Verification items for the finished model (mm, model axes). A direction names the side the tool comes from. Coordinates: 2 decimals unless noted, no trailing zeros. Order: outer loops, then holes, each group sorted by start corner. A loop starts at its lowest first (then second) coordinate and runs counter-clockwise, first axis right, second up. Notation, with made-up numbers: (-13, 3.5) -> (18, 3.5) arc R27 cw to (18, 26.5) -> close; hole circle Ø2 at (19, 27). An arc over 180 degrees is marked (long way). Use CSV: the item, a comma, the result in double quotes. Start each with the question number.
1) Sectioned sample at B-B on z = -66. Record the boundary of the cut face in (x, y) (3 decimals).
2) Tool access check on faces 4 (the cylindrical face through (2.52, 1.93, -47.08)), 5 (the cylindrical face through (-0.069, -1.567, -88.386)), 6 (the flat face through (0, 0, -2.381)). Record the directions out of +Z, -Z, +X, -X, +Y, -Y that give a thin tool (end or side, any length) a straight path to the whole face; none if there is none.
3) Scan lines: line 1 along Z through (x, y) = (3, -2.25); line 2 along Y through (x, z) = (0.25, -23); line 3 along Z through (x, y) = (-0.5, 1.25). Record each from-to range of solid material in increasing order.
4) Go/stop test with flat-tipped pins: pin 1 (0.5 mm diameter, centred on y = -0.5, z = -1, fed in from -X); pin 2 (3 mm diameter, centred on x = -1.5, y = 1.5, fed in from -Z); pin 3 (1 mm diameter, centred on y = 3, z = -62, fed in from -X); pin 4 (1 mm diameter, centred on y = -2.5, z = -83, fed in from -X). Record where each tip stops, or that it passes through.
5) Release check for a two-part mould opening along Y. For faces 1 (the cylindrical face through (-2.302, 0.725, -93.105)), 2 (the flat face through (0.8, 1.37, -1.17)), 3 (the flat face through (0.1, 3.1, -4.763)) record: released by +Y, released by -Y, zero draft, split by the parting line, or undercut.
from build123d import *

# Parameters (mm, degrees)
SKETCH12_R          = 2.413
BOSS_EXTRUDE1_DEPTH = 9.525
CHAMFER1_SIZE       = 0.60325
CHAMFER2_SIZE       = 0.3095625
FILLET1_R           = 0.264583333
CUT_EXTRUDE2_DEPTH  = 2.38125


with BuildPart() as part:
    # Sketch13 → Revolve1 (revolve)
    with BuildSketch(Plane(origin=(0, 0, 0), x_dir=(0, 0, -1), z_dir=(1, 0, 0)), mode=Mode.PRIVATE) as revolve1_sk:
        Polygon((0, 0), (0, 4.7625), (4.7625, 4.7625), (4.7625, 2.936875), (5.715, 2.936875), (5.953125, 3.175), (87.074375, 3.175), (87.3125, 2.936875), (87.3125, 0), align=None)
    revolve(revolve1_sk.sketch.rotate(Axis((0, 0, -87.3125), (0, 0, 1)), 90), axis=Axis((0, 0, -87.3125), (0, 0, 1)))

    # Sketch12 → Boss-Extrude1 (add)
    with BuildSketch(Plane(origin=(0, 0, -87.3125), x_dir=(-1, 0, 0), z_dir=(0, 0, -1))):
        Circle(SKETCH12_R)
    extrude(amount=BOSS_EXTRUDE1_DEPTH)

    # Sketch5 → Cut-Revolve1 (revolve, cut)
    with BuildSketch(Plane(origin=(0, 0, 0), x_dir=(0, 0, -1), z_dir=(1, 0, 0))):
        Polygon((87.3125, 2.413), (90.06205, 2.413), (89.2175, 1.56845), (87.3125, 1.56845), align=None)
    revolve(axis=Axis((0, 0, -87.3125), (0, 0, 1)), mode=Mode.SUBTRACT)

    # Chamfer1
    chamfer1_edges = [part.edges().sort_by_distance(p)[0] for p in [
        (2.413, 0, -96.8375),
    ]]
    chamfer(chamfer1_edges, length=CHAMFER1_SIZE)

    # Chamfer2
    chamfer2_edges = [part.edges().sort_by_distance(p)[0] for p in [
        (4.7625, 0, 0),
    ]]
    chamfer(chamfer2_edges, length=CHAMFER2_SIZE)

    # Fillet1
    fillet1_edges = [part.edges().sort_by_distance(p)[0] for p in [
        (0, -1.56845, -87.3125),
    ]]
    fillet(fillet1_edges, radius=FILLET1_R)

    # Sketch8 → Cut-Extrude2 (cut)
    with BuildSketch(Plane.XY):
        Polygon((1.5875, 0.916543552), (0, 1.833087105), (-1.5875, 0.916543552), (-1.5875, -0.916543552), (0, -1.833087105), (1.5875, -0.916543552), align=None)
    extrude(amount=-CUT_EXTRUDE2_DEPTH, mode=Mode.SUBTRACT)

    # Cut-Extrude4 cone 1 section (through the dimple's axis) → Cut-Extrude4 (revolve, cut)
    with BuildSketch(Plane(origin=(0, 0, 0), x_dir=(0, -1, 0), z_dir=(1, 0, 0))):
        Polygon((0, 0), (1.833087105, 0), (0, 1.833087105), align=None)
    revolve(axis=Axis((0, 0, 0), (0, 0, -1)), mode=Mode.SUBTRACT)


solid = part.part
Answers follow:
1,outline,"circle Ø6.35 at (0, 0)"
2,face 4,"-Z"
2,face 5,"none"
2,face 6,"+Z"
3,line 1,"z = -4.76 to 0"
3,line 2,"y = -3.17 to 3.17"
3,line 3,"z = -96.84 to -2.38"
4,pin 1,"stops at x = -4.76"
4,pin 2,"stops at z = -96.84"
4,pin 3,"stops at x = -1.96"
4,pin 4,"stops at x = -2.47"
5,face 1,"split by the parting line"
5,face 2,"undercut"
5,face 3,"zero draft"
